from build123d import *

# Parameters (mm, degrees)
SKETCH1_W                                     = 123.825
SKETCH1_H                                     = 114.3
PLATE_DEPTH                                   = 3.175
SKETCH2_R                                     = 5.08
FORCE_SENSOR_POST_HOLE_DEPTH                  = 85.317025453
GEARBOX_MOUNT_HOLES_4_CLEARANCE_D             = 3.2639
BEARING_MOUNT_HOLES_4_CLEARANCE_D             = 3.2639
BEARING_MOUNT_HOLES_4_CLEARANCE_DEPTH         = 7.62
BEARING_MOUNT_HOLES_4_CLEARANCE_TIP           = 0.980574487
FORCE_SENSOR_FOUNDATION_HOLES_10_CLEARA_D     = 5.1054
FORCE_SENSOR_FOUNDATION_HOLES_10_CLEARA_DEPTH = 7.62
FORCE_SENSOR_FOUNDATION_HOLES_10_CLEARA_TIP   = 1.533816902
BALL_CASTER_MOUNT_HOLES_4_CLEARANCE_D         = 3.2639
TOP_PLATE_GUIDE_HOLES_10_CLEARANCE_D          = 5.1054


with BuildPart() as part:
    # Sketch1 → Plate (new body)
    with BuildSketch(Plane(origin=(0, 0, 0), x_dir=(1, 0, 0), z_dir=(0, 1, 0))):
        Rectangle(SKETCH1_W, SKETCH1_H)
    extrude(amount=PLATE_DEPTH)

    # Sketch2 → Force Sensor Post Hole (cut, through all)
    with BuildSketch(Plane(origin=(0, 3.175, 0), x_dir=(1, 0, 0), z_dir=(0, 1, 0))):
        with Locations(Location((0, 6.35, 0), (0, 0, 270))):
            Circle(SKETCH2_R)
    extrude(amount=-FORCE_SENSOR_POST_HOLE_DEPTH, mode=Mode.SUBTRACT)

    # Gearbox Mount Holes (#4 clearance) (through all)
    with Locations(Plane(origin=(0, 3.175, 0), x_dir=(1, 0, 0), z_dir=(0, 1, 0))):
        with Locations((-55.4609, -38.1), (-37.0459, -28.575), (-18.6309, -38.1), (-37.0459, -47.625)):
            Hole(GEARBOX_MOUNT_HOLES_4_CLEARANCE_D / 2)

    # Bearing Mount Holes (#4 clearance)
    with Locations(Plane(origin=(0, 3.175, 0), x_dir=(1, 0, 0), z_dir=(0, 1, 0))):
        with Locations((57.15, -24.5745), (30.5816, -51.6255), (30.5816, -24.5745), (57.15, -51.6255)):
            Hole(BEARING_MOUNT_HOLES_4_CLEARANCE_D / 2, depth=BEARING_MOUNT_HOLES_4_CLEARANCE_DEPTH)
            with Locations((0, 0, -(BEARING_MOUNT_HOLES_4_CLEARANCE_DEPTH + BEARING_MOUNT_HOLES_4_CLEARANCE_TIP / 2))):  # 118° drill point
                Cone(0, BEARING_MOUNT_HOLES_4_CLEARANCE_D / 2, BEARING_MOUNT_HOLES_4_CLEARANCE_TIP, mode=Mode.SUBTRACT)

    # Force Sensor Foundation Holes (#10 clearance)
    with Locations(Plane(origin=(0, 3.175, 0), x_dir=(1, 0, 0), z_dir=(0, 1, 0))):
        with Locations((-11.1125, -6.35), (11.1125, 19.05), (-11.1125, 19.05), (11.1125, -6.35), (0, 6.35)):
            Hole(FORCE_SENSOR_FOUNDATION_HOLES_10_CLEARA_D / 2, depth=FORCE_SENSOR_FOUNDATION_HOLES_10_CLEARA_DEPTH)
            with Locations((0, 0, -(FORCE_SENSOR_FOUNDATION_HOLES_10_CLEARA_DEPTH + FORCE_SENSOR_FOUNDATION_HOLES_10_CLEARA_TIP / 2))):  # 118° drill point
                Cone(0, FORCE_SENSOR_FOUNDATION_HOLES_10_CLEARA_D / 2, FORCE_SENSOR_FOUNDATION_HOLES_10_CLEARA_TIP, mode=Mode.SUBTRACT)

    # Ball Caster Mount Holes (#4 clearance) (through all)
    with Locations(Plane(origin=(0, 3.175, 0), x_dir=(1, 0, 0), z_dir=(0, 1, 0))):
        with Locations((-46.2915, 45.339), (-46.2915, 26.416), (-27.3685, 45.339), (46.2915, 45.339), (46.2915, 26.416), (27.3685, 45.339)):
            Hole(BALL_CASTER_MOUNT_HOLES_4_CLEARANCE_D / 2)

    # Top Plate Guide Holes (#10 clearance) (through all)
    with Locations(Plane(origin=(0, 3.175, 0), x_dir=(1, 0, 0), z_dir=(0, 1, 0))):
        with Locations((-46.0375, -12.7), (46.0375, -12.7), (0, 41.275)):
            Hole(TOP_PLATE_GUIDE_HOLES_10_CLEARANCE_D / 2)


solid = part.part
Part model, mm, in its own coordinate system. Round coordinates to 2 decimals unless told otherwise and drop trailing zeros. Loops run counter-clockwise (first coordinate to the right, second up) from the corner with the lowest first, then second, coordinate; pieces in that order, holes last. Notation, with made-up numbers: (3, -30.75) - (58, -30.75) arc R14 ccw to (58, -19.75) - close; hole circle Ø10 at (-34.5, -19.5). An arc over 180 degrees is marked (long way). Answer as a JSON object with one key per item and string values.
Item 1: Pin check, flat tip, straight feed: pin 1 (2 mm diameter, centred on x = 30.58, z = 51.63, fed in from +Y). Stop position of the tip, or through.
Output:
{"pin 1": "through"}
Item 2: Wall check: L1, parallel to Z at x = 45.5, y = 1.7; L2, parallel to X at y = 1.3, z = 25.5; L3, parallel to Z at x = 31, y = 2.95. Give the ranges that are in metal, low to high.
Output:
{"L1": "-57.15 to -46.77, -43.91 to -27.84, -24.99 to 10.2, 15.2 to 57.15", "L2": "-61.91 to 29.24, 31.93 to 55.81, 58.49 to 61.91", "L3": "-57.15 to 23, 26.15 to 50.05, 53.2 to 57.15"}
Item 3: Band-saw the part on D-D on y = 1.95. State how many separate pieces and enclosed holes the cut face has, plus the area to 3 significant figures.
Output:
{"separate pieces": "1", "enclosed holes": "22", "area": "13,800 mm2"}
Item 4: Band-saw the part on B-B on z = 38.1. List the corners of the cut face in (x, y) (1 decimal), plus the area to 3 significant figures.
Output:
{"outline": "(-61.9, 0) - (-57.1, 0) - (-57.1, 3.2) - (-61.9, 3.2) - close; (-53.8, 0) - (-20.3, 0) - (-20.3, 3.2) - (-53.8, 3.2) - close; (-17, 0) - (61.9, 0) - (61.9, 3.2) - (-17, 3.2) - close", "area": "372 mm2"}
Item 5: Band-saw the part on C-C on z = -6.35. List the corners of the cut face in (x, y) (1 decimal), plus the area to 3 significant figures.
Output:
{"outline": "(-61.9, 0) - (-5.1, 0) - (-5.1, 3.2) - (-61.9, 3.2) - close; (5.1, 0) - (61.9, 0) - (61.9, 3.2) - (5.1, 3.2) - close", "area": "361 mm2"}
Item 6: Pull direction X, two halves, no side cores. Call faces 1 (the face through (-28.12, 1.57, -43.89)), 2 (the face through (-1, 3.175, -1)), 3 (the face through (-61.912, 2, 1)): pulls with the +X half, pulls with the -X half, needs draft (parallel to the pull), parting line crosses it, or undercut.
Output:
{"face 1": "undercut", "face 2": "needs draft", "face 3": "pulls with the -X half"}
Item 7: Band-saw the part on A-A on x = 57.15. List the corners of the cut face in (y, z) (3 decimals), plus the area to 3 significant figures.
Output:
{"outline": "(0, -57.15) - (3.175, -57.15) - (3.175, 22.943) - (0, 22.943) - close; (0, 26.206) - (3.175, 26.206) - (3.175, 49.994) - (0, 49.994) - close; (0, 53.257) - (3.175, 53.257) - (3.175, 57.15) - (0, 57.15) - close", "area": "342 mm2"}
